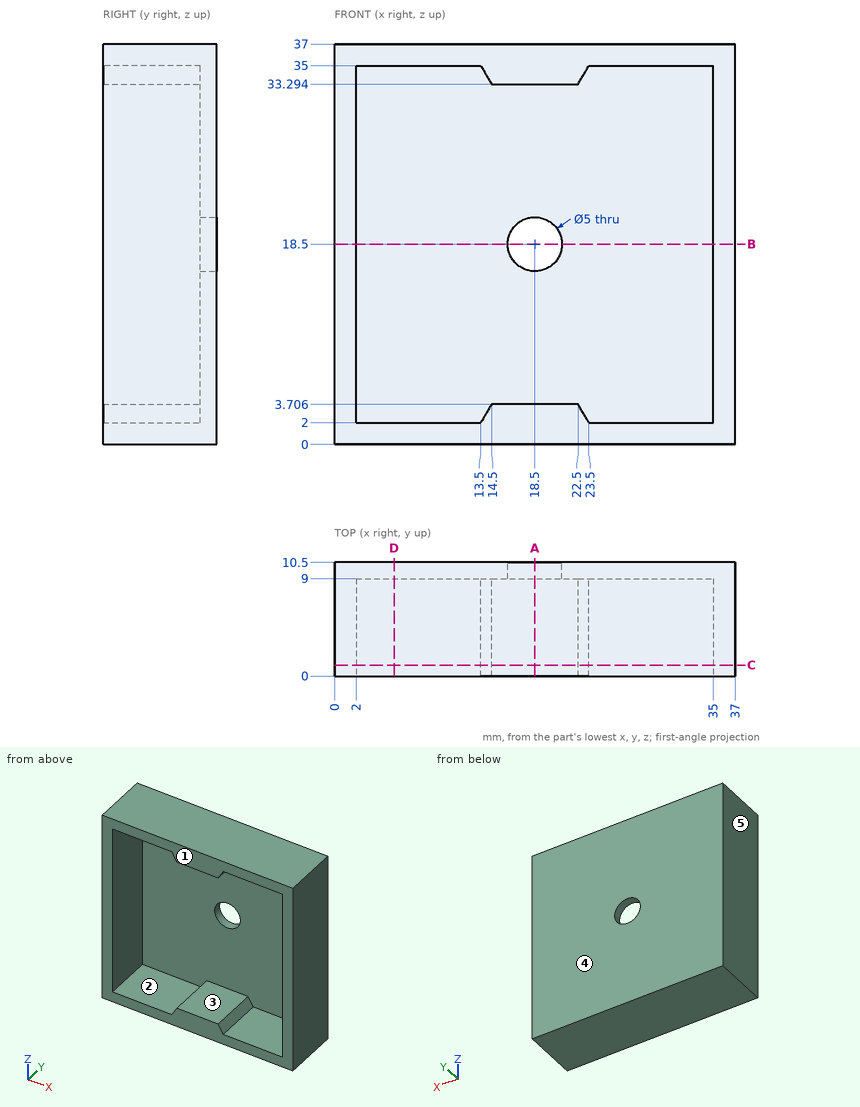
Study the drawing (mm; zero at the part's minimum x, y, z) and answer. A direction names the side the tool comes from. Round coordinates to 2 decimals unless told otherwise and drop trailing zeros. Loops run counter-clockwise (first coordinate to the right, second up) from the corner with the lowest first, then second, coordinate; pieces in that order, holes last.
Q1. Section A-A, the plane x = 18.5 is taken. Determine the outline of the cut face in (y, z).
Q2. Given pin 1 Ø6 at (x, z) = (11.5, 29.5) entering from -Y; pin 2 Ø4 at (x, z) = (18.5, 18.5) entering from +Y, each flat-ended and moving along its own axis, determine where each tip first touches the part or whether it passes through.
Q3. Section C-C, the plane y = 1 is taken. Determine the outline of the cut face in (x, z), then the cut area to 3 significant figures.
Q4. Section B-B, the plane z = 18.5 is taken. Determine the outline of the cut face in (x, y), then the cut area to 3 significant figures.
Q5. For a pull along X with two mould halves and no side action, classify the marked faces 3, 4 and 5 as released by +X, released by -X, zero draft, split by the parting line, or undercut.
Q6. Which of the six approach directions +Z, -Z, +X, -X, +Y, -Y give full straight-line access (tool end or side, diameter ignored) to the marked faces 1 and 2?
Q7. Section D-D, the plane x = 5.5 is taken. Determine the outline of the cut face in (y, z), then the cut area to 3 significant figures.
Q8. Find the intervals of material crossed by line 1 (Z direction, x = 16, y = 1.75); line 2 (Z direction, x = 18.5, y = 9.65); line 3 (X direction, y = 7, z = 11.5), in increasing order.
Completed:
1. outline: (0, 0) - (10.5, 0) - (10.5, 16) - (9, 16) - (9, 3.71) - (0, 3.71) - close; (0, 33.29) - (9, 33.29) - (9, 21) - (10.5, 21) - (10.5, 37) - (0, 37) - close
2. pin 1: stops at y = 9
2. pin 2: passes through
3. outline: (0, 0) - (37, 0) - (37, 37) - (0, 37) - close; hole (2, 2) - (13.5, 2) - (14.5, 3.71) - (22.5, 3.71) - (23.5, 2) - (35, 2) - (35, 35) - (23.5, 35) - (22.5, 33.29) - (14.5, 33.29) - (13.5, 35) - (2, 35) - close
3. area: 311 mm2
4. outline: (0, 0) - (2, 0) - (2, 9) - (16, 9) - (16, 10.5) - (0, 10.5) - close; (21, 9) - (35, 9) - (35, 0) - (37, 0) - (37, 10.5) - (21, 10.5) - close
4. area: 84.0 mm2
5. face 3: undercut
5. face 4: zero draft
5. face 5: released by -X
6. face 1: +Z, -Z, +X, -X, -Y
6. face 2: -Y
7. outline: (0, 0) - (10.5, 0) - (10.5, 37) - (0, 37) - (0, 35) - (9, 35) - (9, 2) - (0, 2) - close
7. area: 91.5 mm2
8. line 1: z = 0 to 3.71, 33.29 to 37
8. line 2: z = 0 to 16, 21 to 37
8. line 3: x = 0 to 2, 35 to 37
